```python
from build123d import *

# Parameters (mm, degrees)
ESQUISSE2_R             = 4
EXTRUSION1_DEPTH        = 3.25
EXTRUSION1_DEPTH_BACK   = 3
ESQUISSE3_OUTSIDE_W     = 24.342
ESQUISSE3_OUTSIDE_H     = 26.972
ESQUISSE3_OUTSIDE_R     = 8.5
ENL_V_MAT_EXTRU_1_DEPTH = 4.25
CHANFREIN1_SIZE         = 1


with BuildPart() as part:
    # Esquisse2 → Extrusion1 (new body, two sides)
    with BuildSketch(Plane(origin=(0, 0, 0), x_dir=(0, 0, -1), z_dir=(1, 0, 0))) as extrusion1_sk:
        Polygon((0, 9.814954576), (-8.5, 4.907477288), (-8.5, -4.907477288), (0, -9.814954576), (8.5, -4.907477288), (8.5, 4.907477288), align=None)
        Circle(ESQUISSE2_R, mode=Mode.SUBTRACT)
    extrude(amount=EXTRUSION1_DEPTH)
    extrude(extrusion1_sk.sketch, amount=-EXTRUSION1_DEPTH_BACK)

    # Esquisse3 outside → Enlèv. mat.-Extru.1 (cut, through all)
    with BuildSketch(Plane(origin=(0, 0, 0), x_dir=(0, 0, -1), z_dir=(1, 0, 0))):
        Rectangle(ESQUISSE3_OUTSIDE_W, ESQUISSE3_OUTSIDE_H)
        Circle(ESQUISSE3_OUTSIDE_R, mode=Mode.SUBTRACT)
    extrude(amount=ENL_V_MAT_EXTRU_1_DEPTH, mode=Mode.SUBTRACT)

    # Esquisse4 → Enlèvement de matière-Révolution1 (revolve, cut)
    with BuildSketch(Plane.XY, mode=Mode.PRIVATE) as enl_vement_de_mati_re_r_volution1_sk:
        with BuildLine():
            Line((-1, 9.814954576), (-3, 9.814954576))
            Line((-3, 9.814954576), (-3, 8.25))
            ThreePointArc((-3, 8.25), (-2.173757557, 9.25453812), (-1, 9.814954576))
        make_face()
    revolve(enl_vement_de_mati_re_r_volution1_sk.sketch.rotate(Axis((0, 0, 0), (-1, 0, 0)), 90), axis=Axis((0, 0, 0), (-1, 0, 0)), mode=Mode.SUBTRACT)  # turned: the seam where the file's is

    # Chanfrein1
    chanfrein1_edges = [part.edges().sort_by_distance(p)[0] for p in [
        (3.25, 0, 4),
        (-3, 0, 4),
    ]]
    chamfer(chanfrein1_edges, length=CHANFREIN1_SIZE)


solid = part.part
```
Part model, mm, in its own coordinate system. A direction names the side the tool comes from. Give positions to 0.01 mm unless a question says otherwise; leave off trailing zeros. Order: outer loops, then holes, each group sorted by start corner. A loop starts at its lowest first (then second) coordinate and runs counter-clockwise, first axis right, second up. Notation, with made-up numbers: M 57,89 L 81,89 A25 ccw 81,118 Z; hole C 67.25,23.5 d4. An arc over 180 degrees is marked long. Use a Markdown table: item, result. Add a question column.
(1) 3-axis set-ups, long thin cutter, end or side, ignore diameter. For faces 1 (the face through (0, -9, 0)), 2 (the face through (0, 4, -8)), 3 (the face through (0, -4, 8)), 4 (the face through (1.602, 7.167, -4.57)): which of +Z, -Z, +X, -X, +Y, -Y reach the whole face in a straight line?
(2) Saw through at A-A, the plane x = -1.5. Give the cut face in (y, z).
(3) Drop flat-ended pins along their axis: P1, Ø3, axis at x = 0, z = -1, coming from the +Y side; P2, Ø4, axis at y = 1, z = -2, coming from the +X side; P3, Ø3, axis at x = 2, z = 5.5, coming from the +Y side. Give the stop position or say it passes through.
(4) Saw through at B-B, the plane x = 0.5. Give the cut face in (y, z).
(5) Probe line 1 along Y through (x, z) = (1.45, 0); line 2 along Z through (x, y) = (-1, 0.5); line 3 along Y through (x, z) = (2.5, -3.5). List the from-to ranges inside material, lowest first. Write a range as [from, to].
Answer key:
| question | item | result |
|---|---|---|
| 1 | face 1 | +X, -Y |
| 1 | face 2 | -Z, +X, +Y |
| 1 | face 3 | +Z, +X, -Y |
| 1 | face 4 | +X |
| 2 | outline | M -9.65,-0.29 L -5.07,-8.21 A9.65 ccw -4.57,-8.5 L 4.57,-8.5 A9.65 ccw 5.07,-8.21 L 9.65,-0.29 A9.65 ccw 9.65,0.29 L 5.07,8.21 A9.65 ccw 4.57,8.5 L -4.57,8.5 A9.65 ccw -5.07,8.21 L -9.65,0.29 A9.65 ccw Z; hole C 0,0 d8 |
| 3 | P1 | y = 9.81 |
| 3 | P2 | x = 2.49 |
| 3 | P3 | y = 7.5 |
| 4 | outline | C 0,0 d17; hole C 0,0 d8 |
| 5 | line 1 | [-8.5, -4], [4, 8.5] |
| 5 | line 2 | [-8.5, -3.97], [3.97, 8.5] |
| 5 | line 3 | [-7.75, -2.41], [2.41, 7.75] |
